For this review, take the finished solid that the model builds, in its own axes (mm). Face numbers are marked on the shaded views. A direction names the side the tool comes from. Coordinates: 2 decimals unless noted, no trailing zeros. Loops run counter-clockwise (first coordinate to the right, second up) from the corner with the lowest first, then second, coordinate; pieces in that order, holes last. Notation, with made-up numbers: (-23, 54.25) - (-16, 54.25) arc R19 ccw to (-16, 74.25) - close; hole circle Ø9 at (-2.75, -9). An arc over 180 degrees is marked (long way). Use one line per item in the form item = value. Start each with the question number.
1. Draft analysis for pull direction Y (two halves, no side actions). For the marked faces 1, 2 and 3, state which applies: +Y half, -Y half, draft (parallel to the pull), parting line (faces both ways), or undercut.
2. Add section A-A on z = -72. Give the boundary of the cut face in (x, y).
3. Add section B-B on x = 10.5. Count the separate pieces of the cut face and the enclosed holes in it, and give its area (3 significant figures).
4. Add section C-C on z = -53. Give the boundary of the cut face in (x, y), and give its area (3 significant figures).
5. Machinability: for the marked faces 4, 5 and 6, which of the approach directions +Z, -Z, +X, -X, +Y, -Y give a long, thin tool a straight path to every point of the face, cutting with its end or side? Answer none if there is none.
6. Add section D-D on x = 6. Give the boundary of the cut face in (y, z), and give its area (3 significant figures).
7. To check wall thickness, follow probe 1 along Y at (x, z) = (9.25, -83.5); probe 2 along X at (y, z) = (-47.5, -20); probe 3 along X at (y, z) = (4, -72). State the ranges of each line that lie inside material, in increasing order.
8. For pin 1 Ø11.5 at (x, z) = (14, -72) entering from +Y; pin 2 Ø14 at (x, y) = (15, -28) entering from -Z; pin 3 Ø6 at (x, y) = (15, -27.5) entering from +Z, all flat-tipped, find the tip position at first contact; note any pin that passes through.
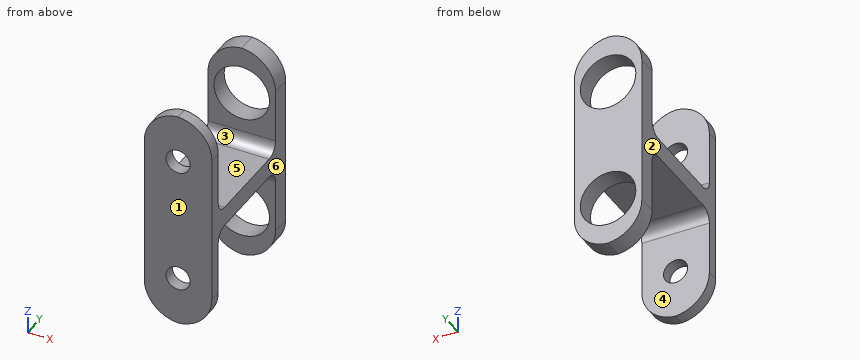
```python
from build123d import *

# Parameters (mm, degrees)
BOSS_EXTRUDE1_DEPTH  = 28
CUT_EXTRUDE1_REACH   = 81.145
SKETCH2_R            = 11.5
CUT_EXTRUDE2_REACH   = 77.558
SKETCH3_R            = 5
FILLET2_R            = 5
FILLET2_OF_MIRROR2_R = 5
FILLET3_R            = 15


with BuildPart() as part:
    # Sketch1 → Boss-Extrude1 (new body)
    with BuildSketch(Plane(origin=(0, 0, 0), x_dir=(0, 0, -1), z_dir=(1, 0, 0))):
        Polygon((0, 0), (42, 0), (42, -45), (0, -45), (0, -50), (46, -50), (46, 8), (0, 8), align=None)
    boss_extrude1 = extrude(amount=BOSS_EXTRUDE1_DEPTH)

    # Sketch2 → Cut-Extrude1 (cut, up to next)
    with BuildSketch(Plane(origin=(0, 8, 0), x_dir=(1, 0, 0), z_dir=(0, 1, 0)), mode=Mode.PRIVATE) as cut_extrude1_sk1:
        with Locations(Location((14, 20, 0), (0, 0, 270))):
            Circle(SKETCH2_R)
    cut_extrude1_tool1 = extrude(cut_extrude1_sk1.sketch, amount=-CUT_EXTRUDE1_REACH, mode=Mode.PRIVATE) & part.part
    cut_extrude1 = cut_extrude1_tool1.solids().sort_by_distance((14, 8, -20))[0]
    add(cut_extrude1, mode=Mode.SUBTRACT)

    # Sketch3 → Cut-Extrude2 (cut, up to next)
    with BuildSketch(Plane(origin=(0, -45, 0), x_dir=(1, 0, 0), z_dir=(0, 1, 0)), mode=Mode.PRIVATE) as cut_extrude2_sk1:
        with Locations(Location((14, 20, 0), (0, 0, 270))):
            Circle(SKETCH3_R)
    cut_extrude2_tool1 = extrude(cut_extrude2_sk1.sketch, amount=-CUT_EXTRUDE2_REACH, mode=Mode.PRIVATE) & part.part
    cut_extrude2 = cut_extrude2_tool1.solids().sort_by_distance((14, -45, -20))[0]
    add(cut_extrude2, mode=Mode.SUBTRACT)

    # Fillet2
    fillet2_edges = [part.edges().sort_by_distance(p)[0] for p in [
        (14, -45, -42),
        (14, 0, -42),
    ]]
    fillet(fillet2_edges, radius=FILLET2_R)

    # Mirror2: Boss-Extrude1, Cut-Extrude1, Cut-Extrude2 across plane
    add(boss_extrude1.mirror(Plane(origin=(28, -50, -46), x_dir=(1, 0, 0), z_dir=(0, 0, 1))))
    add(cut_extrude1.mirror(Plane(origin=(28, -50, -46), x_dir=(1, 0, 0), z_dir=(0, 0, 1))), mode=Mode.SUBTRACT)
    add(cut_extrude2.mirror(Plane(origin=(28, -50, -46), x_dir=(1, 0, 0), z_dir=(0, 0, 1))), mode=Mode.SUBTRACT)

    # Fillet2 of Mirror2
    fillet2_of_mirror2_edges = [part.edges().sort_by_distance(p)[0] for p in [
        (14, -45, -50),
        (14, 0, -50),
    ]]
    fillet(fillet2_of_mirror2_edges, radius=FILLET2_OF_MIRROR2_R)

    # Fillet3
    # the kernel refuses this fillet: 15 mm, written as the material it takes off along each edge
    with BuildSketch(Plane(origin=(0, -7.5, 0), x_dir=(0, 0, -1), z_dir=(0, -1, 0)), Plane(origin=(28, -7.5, 0), x_dir=(-1, 0, 0), z_dir=(0, -1, 0))) as fillet3_piece_1:
        with BuildLine():
            CenterArc((FILLET3_R, FILLET3_R), FILLET3_R, 180, 90)
            Line((0, FILLET3_R), (0, 0))
            Line((0, 0), (FILLET3_R, 0))
        make_face()
    extrude(amount=80, mode=Mode.SUBTRACT)
    with BuildSketch(Plane(origin=(0, 45.5, 0), x_dir=(0, 0, -1), z_dir=(0, -1, 0)), Plane(origin=(28, 45.5, 0), x_dir=(-1, 0, 0), z_dir=(0, -1, 0))) as fillet3_piece_2:
        with BuildLine():
            CenterArc((FILLET3_R, FILLET3_R), FILLET3_R, 180, 90)
            Line((0, FILLET3_R), (0, 0))
            Line((0, 0), (FILLET3_R, 0))
        make_face()
    extrude(amount=83, mode=Mode.SUBTRACT)
    with BuildSketch(Plane(origin=(0, 45.5, -92), x_dir=(0, 0, 1), z_dir=(0, -1, 0)), Plane(origin=(28, 45.5, -92), x_dir=(-1, 0, 0), z_dir=(0, -1, 0))) as fillet3_piece_3:
        with BuildLine():
            CenterArc((FILLET3_R, -FILLET3_R), FILLET3_R, 90, 90)
            Line((0, -FILLET3_R), (0, 0))
            Line((0, 0), (FILLET3_R, 0))
        make_face()
    extrude(amount=83, mode=Mode.SUBTRACT)
    with BuildSketch(Plane(origin=(0, -7.5, -92), x_dir=(0, 0, 1), z_dir=(0, -1, 0)), Plane(origin=(28, -7.5, -92), x_dir=(-1, 0, 0), z_dir=(0, -1, 0))) as fillet3_piece_4:
        with BuildLine():
            CenterArc((FILLET3_R, -FILLET3_R), FILLET3_R, 90, 90)
            Line((0, -FILLET3_R), (0, 0))
            Line((0, 0), (FILLET3_R, 0))
        make_face()
    extrude(amount=80, mode=Mode.SUBTRACT)


solid = part.part
```
Conclusion:
q1.face_1 = -Y half
q1.face_2 = draft
q1.face_3 = undercut
q2.outline = (0, -50) - (9, -50) - (9, -45) - (0, -45) - close; (0, 0) - (2.5, 0) - (2.5, 8) - (0, 8) - close; (19, -50) - (28, -50) - (28, -45) - (19, -45) - close; (25.5, 0) - (28, 0) - (28, 8) - (25.5, 8) - close
q3.separate_pieces = 5
q3.enclosed_holes = 0
q3.area = 1,140 mm^2
q4.outline = (0, -50) - (28, -50) - (28, -44.58) - (0, -44.58) - close; (0, -0.42) - (28, -0.42) - (28, 8) - (0, 8) - close
q4.area = 387 mm^2
q5.face_4 = -Z, +X, -X
q5.face_5 = +Z, +X, -X
q5.face_6 = +Z, -Z, +X, +Y, -Y
q6.outline = (-50, -89) - (-45, -89) - (-45, -55) arc R5 cw to (-40, -50) - (-5, -50) arc R5 cw to (0, -55) - (0, -63.74) - (8, -63.74) - (8, -28.26) - (0, -28.26) - (0, -37) arc R5 cw to (-5, -42) - (-40, -42) arc R5 cw to (-45, -37) - (-45, -3) - (-50, -3) - close; (0, -89) - (8, -89) - (8, -80.26) - (0, -80.26) - close; (0, -11.74) - (8, -11.74) - (8, -3) - (0, -3) - close
q6.area = 1,240 mm^2
q7.probe_1 = -50 to -45, 0 to 8
q7.probe_2 = 0 to 9, 19 to 28
q7.probe_3 = 0 to 2.5, 25.5 to 28
q8.pin_1 = -45
q8.pin_2 = -50
q8.pin_3 = -42
